Can you work these out from the model? Positions are in its coordinate system, mm. A direction names the side the tool comes from. Give positions to 0.01 mm unless a question says otherwise; leave off trailing zeros. Order: outer loops, then holes, each group sorted by start corner. A loop starts at its lowest first (then second) coordinate and runs counter-clockwise, first axis right, second up. Notation, with made-up numbers: (36, 74) -> (92, 74) arc R25 ccw to (92, 112) -> close; hole circle Ø3 at (54, 27). An arc over 180 degrees is marked (long way). Answer as a JSON object with one key per item and string values.
```python
from build123d import *

# Parameters (mm, degrees)
SKETCH1_R      = 1.05
SKETCH1_R_2    = 4
SKETCH1_R_3    = 1.6
EXTRUDE1_DEPTH = 3
FILLET1_R      = 3


with BuildPart() as part:
    # Sketch1 → Extrude1 (new body)
    with BuildSketch(Plane.XY):
        Polygon((-83.5, 74.115427319), (25.779226165, 74.115427319), (102.5, 38.33994294), (102.5, 11.115427319), (-6.779226165, 11.115427319), (-83.5, 46.890911697), align=None)
        with Locations((-79.25, 69.915427319)):
            Circle(SKETCH1_R, mode=Mode.SUBTRACT)
        with Locations((-11.75, 69.915427319)):
            Circle(SKETCH1_R, mode=Mode.SUBTRACT)
        with Locations((0, 16.201854058)):
            Circle(SKETCH1_R_2, mode=Mode.SUBTRACT)
        with Locations((95, 16.201854058)):
            Circle(SKETCH1_R_2, mode=Mode.SUBTRACT)
        with Locations((95, 27)):
            Circle(SKETCH1_R_3, mode=Mode.SUBTRACT)
        with Locations((95, 34.5)):
            Circle(SKETCH1_R_3, mode=Mode.SUBTRACT)
        with Locations((0, 34.5)):
            Circle(SKETCH1_R_3, mode=Mode.SUBTRACT)
        with Locations((0, 27)):
            Circle(SKETCH1_R_3, mode=Mode.SUBTRACT)
        Polygon((-63.5, 54.115427319), (-13.5, 54.115427319), (-13.5, 30.800044411), align=None, mode=Mode.SUBTRACT)
        Polygon((16.5, 61.891732757), (16.5, 31.115427319), (82.5, 31.115427319), align=None, mode=Mode.SUBTRACT)
    extrude(amount=EXTRUDE1_DEPTH)

    # Fillet1
    fillet1_edges = [part.edges().sort_by_distance(p)[0] for p in [
        (82.5, 31.115427319, 1.5),
        (16.5, 61.891732757, 1.5),
        (16.5, 31.115427319, 1.5),
    ]]
    fillet(fillet1_edges, radius=FILLET1_R)


solid = part.part
```
1. If we mould it in two halves opening along X, with no side actions, what happens to faces 3 (the face through (63.6, 56.48, 1.48)), 4 (the face through (11, 43, 3)), 5 (the face through (17.924, 59.735, 1.521))? For each: +X half, -X half, draft (parallel to the pull), parting line (faces both ways), or undercut.
Worked answers:
{"face 3": "+X half", "face 4": "draft", "face 5": "undercut"}
2. Will these pins go through, and if not, where does the flat tip stop? pin 1 Ø1.5 at (y, z) = (41, 2) entering from -X; pin 2 Ø0.9 at (x, z) = (42, 1) entering from +Y; pin 3 Ø0.9 at (x, z) = (-37, 1) entering from -Y.
Worked answers:
{"pin 1": "x = -72.48", "pin 2": "y = 66.76", "pin 3": "y = 25"}
3. If we section it at B-B on z = 1.45: Count the separate pieces of the cut face and the enclosed holes in it, then the cut area to 3 significant figures.
Worked answers:
{"separate pieces": "1", "enclosed holes": "10", "area": "7,270 mm²"}
4. For faces 1 (the face through (-30, 74.115, 1)), 2 (the face through (-38.15, 42.295, 1.479)), which set-ups out of +Z, -Z, +X, -X, +Y, -Y let a thin tool reach every point of the face, with its end or its side?
Worked answers:
{"face 1": "+Z, -Z, +X, -X, +Y", "face 2": "+Z, -Z"}
5. Please list where these lines run through material, in increasing order: L1, parallel to Y at x = 0, z = 1.35; L2, parallel to X at y = 40.5, z = 2.5; L3, parallel to X at y = 69, z = 2.8.
Worked answers:
{"L1": "11.12 to 12.2, 20.2 to 25.4, 28.6 to 32.9, 36.1 to 74.12", "L2": "-69.79 to -34.3, -13.5 to 16.5, 62.37 to 97.87", "L3": "-83.5 to -79.76, -78.74 to -12.26, -11.24 to 36.75"}
6. If we section it at D-D on y = 22.5: Please give me the cut outline in (x, z).
Worked answers:
{"outline": "(-31.19, 0) -> (102.5, 0) -> (102.5, 3) -> (-31.19, 3) -> close"}
7. If we section it at A-A on x = 0: Please give me the cut outline in (y, z).
Worked answers:
{"outline": "(11.12, 0) -> (12.2, 0) -> (12.2, 3) -> (11.12, 3) -> close; (20.2, 0) -> (25.4, 0) -> (25.4, 3) -> (20.2, 3) -> close; (28.6, 0) -> (32.9, 0) -> (32.9, 3) -> (28.6, 3) -> close; (36.1, 0) -> (74.12, 0) -> (74.12, 3) -> (36.1, 3) -> close"}
8. If we section it at C-C on x = 95: Please give me the cut outline in (y, z).
Worked answers:
{"outline": "(11.12, 0) -> (12.2, 0) -> (12.2, 3) -> (11.12, 3) -> close; (20.2, 0) -> (25.4, 0) -> (25.4, 3) -> (20.2, 3) -> close; (28.6, 0) -> (32.9, 0) -> (32.9, 3) -> (28.6, 3) -> close; (36.1, 0) -> (41.84, 0) -> (41.84, 3) -> (36.1, 3) -> close"}
